from build123d import *

# Parameters (mm, degrees)
F0_R     = 5
F1_DEPTH = 64
F4_W     = 18.964292
F4_H     = 17.682846
F4_W_2   = 5
F4_H_2   = 14.245734
F5_DEPTH = 10
F6_W     = 13
F6_H     = 2
F7_DEPTH = 12.5
F8_R     = 4
F9_DEPTH = 8


with BuildPart() as f1:
    # F0 (on Right) → F1 (new body)
    with BuildSketch(Plane.YZ):
        Circle(F0_R)
    extrude(amount=F1_DEPTH)

    # F2 (on Front) → F3 (revolve, cut)
    with BuildSketch(Plane.XZ):
        Polygon((10, 6.419506), (10, 3), (38, 3), (38, 4.927536), (40, 4.927536), (40, 3), (64, 3), (64, 6.419506), align=None)
    revolve(axis=Axis((28.04348, 0, 0), (1, 0, 0)), mode=Mode.SUBTRACT)

    # F4 (on face) → F5 (cut)
    with BuildSketch(Plane.YZ.offset(64)):
        Rectangle(F4_W, F4_H)
        Rectangle(F4_W_2, F4_H_2, mode=Mode.SUBTRACT)
    extrude(amount=-F5_DEPTH, mode=Mode.SUBTRACT)

    # F6 (on Top) → F7 (cut, symmetric)
    with BuildSketch(Plane.XY):
        Rectangle(F6_W, F6_H)
        with BuildLine():
            Line((6.5, 1), (6.5, -1))
            ThreePointArc((6.5, -1), (7.5, 0), (6.5, 1))
        make_face()
    extrude(amount=F7_DEPTH, both=True, mode=Mode.SUBTRACT)

    # F8 (on face) → F9 (cut)
    with BuildSketch(Plane(origin=(0, 0, 0), x_dir=(0, -1, 0), z_dir=(-1, 0, 0))):
        Circle(F8_R)
    extrude(amount=-F9_DEPTH, mode=Mode.SUBTRACT)


solid = f1.part
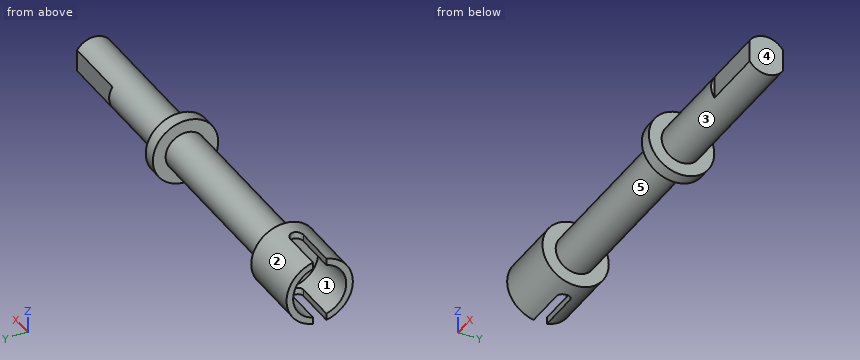
Read the model definition and answer for the solid it produces. Units are mm, in the model's axes. Face numbers are marked on the shaded views. A direction names the side the tool comes from. Coordinates: 2 decimals unless noted, no trailing zeros. Loops run counter-clockwise (first coordinate to the right, second up) from the corner with the lowest first, then second, coordinate; pieces in that order, holes last.
Q1. The part is cut by section A-A on z = 0. Write down the section's boundary in (x, y).
Q2. The part is cut by section D-D on x = 59. Write down the section's boundary in (y, z).
Q3. The part is cut by section B-B on y = 0. Write down the section's boundary in (x, z), and give its area (3 significant figures).
Q4. The mould has two halves that part along X. Classify the marked faces 3, 4 and 5: +X half, -X half, draft (parallel to the pull), parting line (faces both ways), or undercut.
Q5. Each of these flat-tipped pins is pushed along its axis until it touches: pin 1 Ø3.5 at (x, z) = (57, 0.5) entering from +Y; pin 2 Ø1.5 at (x, y) = (40.5, 0.5) entering from +Z; pin 3 Ø3 at (x, z) = (12, 0.5) entering from +Y. Where does it stop, or does it pass through?
Q6. Consider probe 1 along X at (y, z) = (2.25, 3); probe 2 along X at (y, z) = (3.5, -3); probe 3 along X at (y, z) = (-1, 2.25). Determine where each line is inside the solid, lowest interval first.
Q7. Which of the six approach directions +Z, -Z, +X, -X, +Y, -Y give full straight-line access (tool end or side, diameter ignored) to the marked faces 1 and 2?
Q8. The part is cut by section C-C on x = 51.5. Write down the section's boundary in (y, z), and give its area (3 significant figures).
Results below:
1. outline: (0, -5) - (10, -5) - (10, -3) - (38, -3) - (38, -4.93) - (40, -4.93) - (40, -3) - (54, -3) - (54, -2.5) - (64, -2.5) - (64, 2.5) - (54, 2.5) - (54, 3) - (40, 3) - (40, 4.93) - (38, 4.93) - (38, 3) - (10, 3) - (10, 5) - (0, 5) - (0, 4) - (8, 4) - (8, -4) - (0, -4) - close
2. outline: (-2.5, -1.66) arc R3 ccw to (2.5, -1.66) - (2.5, 1.66) arc R3 ccw to (-2.5, 1.66) - close
3. outline: (7.5, -5) - (10, -5) - (10, -3) - (38, -3) - (38, -4.93) - (40, -4.93) - (40, -3) - (64, -3) - (64, 3) - (40, 3) - (40, 4.93) - (38, 4.93) - (38, 3) - (10, 3) - (10, 5) - (7.5, 5) - (7.5, 4) - (8, 4) - (8, -4) - (7.5, -4) - close
3. area: 353 mm2
4. face 3: draft
4. face 4: +X half
4. face 5: undercut
5. pin 1: stops at y = 2.5
5. pin 2: stops at z = 4.93
5. pin 3: stops at y = 3
6. probe 1: x = 8 to 10, 38 to 40
6. probe 2: x = 0 to 10, 38 to 40
6. probe 3: x = 8 to 64
7. face 1: -X
7. face 2: +X, -X
8. outline: circle Ø6 at (0, 0)
8. area: 28.3 mm2
